Autodesk Inventor part; units mm, degrees
ref_plane "YZ Plane" through (0, 0, 0) normal (1, 0, 0) x (0, 1, 0)
ref_plane "XZ Plane" through (0, 0, 0) normal (0, 1, 0) x (-1, 0, 0)
ref_plane "XY Plane" through (0, 0, 0) normal (0, 0, 1) x (1, 0, 0)
sketch "Sketch1" plane through (0, 0, 0) normal (0, 1, 0) x (-1, 0, 0)
  circle A0 centre (-0.5725, 7.3819) radius 2.25
  circle A1 centre (-0.5725, -4.6791) radius 2.25
  line L0 (2.9275, 11.3819) -> (-4.0725, 11.3819)
  line L1 (-4.0725, 11.3819) -> (-4.0725, -8.6181)
  line L2 (-4.0725, -8.6181) -> (2.9275, -8.6181)
  line L3 (2.9275, -8.6181) -> (2.9275, 11.3819)
  point P0 (0, 0)
  dimension "d0" = 4.5
  dimension "d1" = 4.5
  dimension "d2" = 12.061
  dimension "d3" = 7
  dimension "d4" = 3.5
  dimension "d5" = 20
  dimension "d6" = 4
extrude "Extrusion1" add sketch "Sketch1" along normal blind 10
fillet "Fillet1" radius 2 4 edges at (-2.9275, 5, 11.3819) (4.0725, 5, 11.3819) (4.0725, 5, -8.6181) (-2.9275, 5, -8.6181)
properties part number "Aparter"
Check sheet for the modelled part. Datum: model origin and axes. Units: mm. Give positions to 0.01 mm unless a question says otherwise; leave off trailing zeros. Write each loop counter-clockwise with the first axis right and the second up, starting at its lowest first coordinate (ties: lowest second). Pieces come first, ordered by that corner, then holes. Notation, with made-up numbers: (14, 76.25) -> (21, 76.25) arc R18 cw to (21, 85.25) -> close; hole circle Ø1 at (-20, 63). An arc over 180 degrees is marked (long way). Use CSV: the item, a comma, the result in double quotes. Start each with the question number.
Q1. Cross-section at C-C on y = 9. Enter the section's corners in (x, z).
Q2. Cross-section at A-A on z = 5.5. Enter the section's corners in (x, y).
Q3. Release check for a two-part mould opening along X. For faces 1 (the cylindrical face through (0.87, 4.93, -6.91)), 2 (the flat face through (4.072, 5, 1)), 3 (the cylindrical face through (-2.36, 5.07, 10.78)), 4 (the flat face through (1, 5, 11.382)) record: +X half, -X half, draft (parallel to the pull), parting line (faces both ways), or undercut.
Q4. Depth check by flat-ended pin: P1, Ø1, axis at x = 1, z = -6, coming from the -Y side. Enter the tip coordinate at first touch or a pass-through.
Q5. Cross-section at D-D on z = 8.5. Enter the section's corners in (x, y), and give its area (3 significant figures).
Q6. Cross-section at B-B on x = 2.5. Enter the section's corners in (y, z).
Q7. Scan lines: line 1 along X through (y, z) = (8, 7.5); line 2 along Z through (x, y) = (2.5, 8); line 3 along Z through (x, y) = (-0.5, 0.75). Record each from-to range of solid material in increasing order.
Working result:
1,outline,"(-2.93, -6.62) arc R2 ccw to (-0.93, -8.62) -> (2.07, -8.62) arc R2 ccw to (4.07, -6.62) -> (4.07, 9.38) arc R2 ccw to (2.07, 11.38) -> (-0.93, 11.38) arc R2 ccw to (-2.93, 9.38) -> close; hole circle Ø4.5 at (0.57, -4.68); hole circle Ø4.5 at (0.57, 7.38)"
2,outline,"(-2.93, 0) -> (-0.66, 0) -> (-0.66, 10) -> (-2.93, 10) -> close; (1.81, 0) -> (4.07, 0) -> (4.07, 10) -> (1.81, 10) -> close"
3,face 1,"undercut"
3,face 2,"+X half"
3,face 3,"-X half"
3,face 4,"draft"
4,P1,"passes through"
5,outline,"(-2.93, 0) -> (-1.38, 0) -> (-1.38, 10) -> (-2.93, 10) -> close; (2.53, 0) -> (4.07, 0) -> (4.07, 10) -> (2.53, 10) -> close"
5,area,"30.9 mm^2"
6,outline,"(0, -8.57) -> (10, -8.57) -> (10, -5.84) -> (0, -5.84) -> close; (0, -3.52) -> (10, -3.52) -> (10, 6.22) -> (0, 6.22) -> close; (0, 8.54) -> (10, 8.54) -> (10, 11.34) -> (0, 11.34) -> close"
7,line 1,"x = -2.93 to -1.67, 2.82 to 4.07"
7,line 2,"z = -8.57 to -5.84, -3.52 to 6.22, 8.54 to 11.34"
7,line 3,"z = -8.62 to -6.66, -2.7 to 5.4, 9.36 to 11.38"
